Input: part model. Units: mm. Frame: model coordinates. A direction names the side the tool comes from. Give positions to 0.01 mm unless a question says otherwise; leave off trailing zeros. Loops run counter-clockwise (first coordinate to the right, second up) from the corner with the lowest first, then second, coordinate; pieces in that order, holes last. Notation, with made-up numbers: (1.25, -10) -> (13.25, -10) arc R24 cw to (13.25, 22) -> close; hole circle Ø4 at (-22, 10). An arc over 180 degrees is marked (long way). Answer as a JSON object with one key per item and string values.
```python
from build123d import *

# Parameters (mm, degrees)
SALIENTE_EXTRUIR1_DEPTH      = 100
SALIENTE_EXTRUIR1_DEPTH_BACK = 100
CROQUIS1_R                   = 120
SALIENTE_EXTRUIR4_DEPTH      = 115
SALIENTE_EXTRUIR4_DEPTH_BACK = 115
CROQUIS3_R                   = 275
CROQUIS3_R_2                 = 115
REDONDEO1_R                  = 40
REDONDEO2_R                  = 10
REDONDEO3_R                  = 10


with BuildPart() as part:
    # Croquis1 → Saliente-Extruir1 (new, two sides: drawn at the far end of the back side and taken through both)
    with BuildSketch(Plane(origin=(0, 0, 0), x_dir=(1, 0, 0), z_dir=(0, 1, 0)).offset(-SALIENTE_EXTRUIR1_DEPTH_BACK)):
        with Locations(Location((0, 0, 0), (0, 0, 270))):
            Circle(CROQUIS1_R)
    extrude(amount=SALIENTE_EXTRUIR1_DEPTH + SALIENTE_EXTRUIR1_DEPTH_BACK)

    # Croquis3 → Saliente-Extruir4 (add, two sides: drawn at the far end of the back side and taken through both)
    with BuildSketch(Plane(origin=(0, 0, 0), x_dir=(1, 0, 0), z_dir=(0, 1, 0)).offset(-SALIENTE_EXTRUIR4_DEPTH_BACK)):
        with Locations(Location((0, 0, 0), (0, 0, 270))):
            Circle(CROQUIS3_R)
        with Locations(Location((0, 0, 0), (0, 0, 270))):
            Circle(CROQUIS3_R_2, mode=Mode.SUBTRACT)
    extrude(amount=SALIENTE_EXTRUIR4_DEPTH + SALIENTE_EXTRUIR4_DEPTH_BACK)

    # Redondeo1
    redondeo1_edges = [part.edges().sort_by_distance(p)[0] for p in [
        (0, 115, -275),
        (0, -115, -275),
    ]]
    fillet(redondeo1_edges, radius=REDONDEO1_R)

    # Redondeo2
    redondeo2_edges = [part.edges().sort_by_distance(p)[0] for p in [
        (0, -115, -115),
    ]]
    fillet(redondeo2_edges, radius=REDONDEO2_R)

    # Redondeo3
    redondeo3_edges = [part.edges().sort_by_distance(p)[0] for p in [
        (0, 115, -115),
    ]]
    fillet(redondeo3_edges, radius=REDONDEO3_R)


solid = part.part
```
Q1. Access query for faces 4 (the flat face through (2, 100, -2)), 5 (the flat face through (2, -100, -2)), 6 (the flat face through (-101, -115, 101)). Directions: +Z, -Z, +X, -X, +Y, -Y. A direction counts if a zero-diameter tool reaches every point of the face in a straight line with its end or side. Return the directions, or none.
Evaluation:
{"face 4": "+Y", "face 5": "-Y", "face 6": "+Z, -Z, +X, -X, -Y"}
Q2. Section C-C, the plane y = -86.5. Return the cut outline in (x, z).
Evaluation:
{"outline": "circle Ø546.62 at (0, 0)"}
Q3. Ray query, line 1 along X through (y, z) = (103.25, 0); line 2 along X through (y, z) = (102, 0); line 3 along Y through (x, z) = (21, 107.5). Return the intervals inside material, ascending.
Evaluation:
{"line 1": "x = -263.32 to -115, 115 to 263.32", "line 2": "x = -264.51 to -115, 115 to 264.51", "line 3": "y = -100 to 100"}
Q4. Section A-A, the plane z = 0. Return the cut outline in (x, y), then the cut area to 3 significant figures.
Evaluation:
{"outline": "(-275, -75) arc R40 ccw to (-235, -115) -> (-125, -115) arc R10 ccw to (-115, -105) -> (-115, -100) -> (115, -100) -> (115, -105) arc R10 ccw to (125, -115) -> (235, -115) arc R40 ccw to (275, -75) -> (275, 75) arc R40 ccw to (235, 115) -> (125, 115) arc R10 ccw to (115, 105) -> (115, 100) -> (-115, 100) -> (-115, 105) arc R10 ccw to (-125, 115) -> (-235, 115) arc R40 ccw to (-275, 75) -> close", "area": "118,000 mm2"}
Q5. Draft query along X for faces 1 (the flat face through (-101, 115, 101)), 2 (the cylindrical face through (82.6, -1, 262.3)), 3 (the cylindrical face through (-112.265, -102.535, -24.93)). Return one class per face: +X half, -X half, draft (parallel to the pull), parting line (faces both ways), or undercut.
Evaluation:
{"face 1": "draft", "face 2": "parting line", "face 3": "undercut"}
Q6. Pin query (flat end, axial travel): pin 1 (6 mm diameter, centred on x = -188, z = -160.5, fed in from -Y); pin 2 (4 mm diameter, centred on x = 187, z = 198, fed in from -Y); pin 3 (3 mm diameter, centred on y = 73, z = 175.5, fed in from +X). Return the tip coordinate at first contact, or that it passes through.
Evaluation:
{"pin 1": "stops at y = -113.93", "pin 2": "stops at y = -93.72", "pin 3": "stops at x = 212.95"}
Q7. Section B-B, the plane y = 40.5. Return the cut outline in (x, z), then the cut area to 3 significant figures.
Evaluation:
{"outline": "circle Ø550 at (0, 0)", "area": "238,000 mm2"}
